The model under review builds one solid part; all positions refer to its coordinate system, in mm. Give positions to 0.01 mm unless a question says otherwise; leave off trailing zeros. Order: outer loops, then holes, each group sorted by start corner. A loop starts at its lowest first (then second) coordinate and runs counter-clockwise, first axis right, second up. Notation, with made-up numbers: (40.5, -20) -> (45.5, -20) arc R18 ccw to (45.5, 9) -> close; hole circle Ø11 at (61, -6). An arc over 180 degrees is marked (long way). Use one line per item in the form item = value.
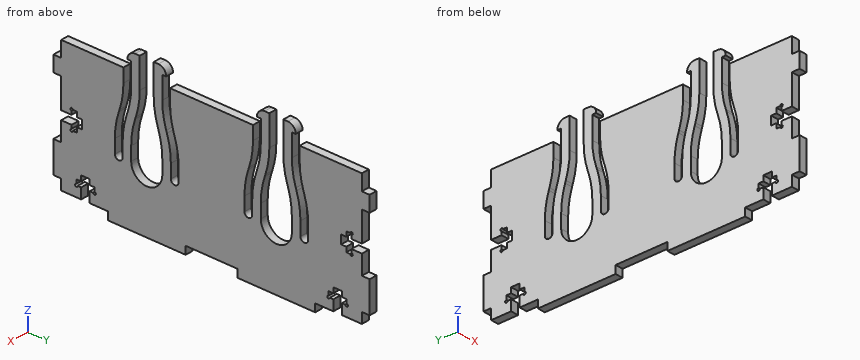
```python
from build123d import *

# Parameters (mm, degrees)
F0_W     = 3
F0_H     = 6
F0_H_2   = 12
F0_W_2   = 30
F0_H_3   = 3
F1_DEPTH = 1.5


# Not quite as in the source:
# - a feature names something its author has since deleted; it is built from what else it names


with BuildPart() as f1:
    # F0 (on Right) → F1 (new body, symmetric)
    with BuildSketch(Plane.YZ):
        with BuildLine():
            Line((50.3, -25), (58, -25))
            Line((58, -25), (58, -21))
            Line((58, -21), (58, -9))
            Line((58, -9), (58, -1.65))
            Line((58, -1.65), (54, -1.65))
            Line((54, -1.65), (54, -3))
            ThreePointArc((54, -3), (54.3535533906, -3.1464466094), (54.5, -3.5))
            ThreePointArc((54.5, -3.5), (54, -4), (53.5, -3.5))
            Line((53.5, -3.5), (52, -3.5))
            Line((52, -3.5), (52, -1.65))
            Line((52, -1.65), (50, -1.65))
            Line((50, -1.65), (50, 1.65))
            Line((50, 1.65), (52, 1.65))
            Line((52, 1.65), (52, 3.5))
            Line((52, 3.5), (53.5, 3.5))
            ThreePointArc((53.5, 3.5), (54, 4), (54.5, 3.5))
            ThreePointArc((54.5, 3.5), (54.3535533906, 3.1464466094), (54, 3))
            Line((54, 3), (54, 1.65))
            Line((54, 1.65), (58, 1.65))
            Line((58, 1.65), (58, 13))
            Line((58, 13), (58, 19))
            Line((58, 19), (58, 25))
            Line((58, 25), (34, 25))
            Line((34, 25), (34, 19.8221099082))
            ThreePointArc((34, 19.8221099082), (34.3801942596, 15.0611112835), (35.5111405269, 10.4207862821))
            Line((35.5111405269, 10.4207862821), (35.7888594731, 9.5792137179))
            ThreePointArc((35.7888594731, 9.5792137179), (36.9198057404, 4.9388887165), (37.3, 0.1778900918))
            Line((37.3, 0.1778900918), (37.3, -5))
            ThreePointArc((37.3, -5), (35.8, -6.5), (34.3, -5))
            Line((34.3, -5), (34.3, 0.1778900918))
            ThreePointArc((34.3, 0.1778900918), (33.9198057404, 4.9388887165), (32.7888594731, 9.5792137179))
            Line((32.7888594731, 9.5792137179), (32.5111405269, 10.4207862821))
            ThreePointArc((32.5111405269, 10.4207862821), (31.3801942596, 15.0611112835), (31, 19.8221099082))
            Line((31, 19.8221099082), (31, 25))
            Line((31, 25), (27.7, 25))
            Line((27.7, 25), (27.7, 19.8221099082))
            ThreePointArc((27.7, 19.8221099082), (28.0801942596, 15.0611112835), (29.2111405269, 10.4207862821))
            Line((29.2111405269, 10.4207862821), (29.4888594731, 9.5792137179))
            ThreePointArc((29.4888594731, 9.5792137179), (30.6198057404, 4.9388887165), (31, 0.1778900918))
            Line((31, 0.1778900918), (31, -5))
            ThreePointArc((31, -5), (25, -11), (19, -5))
            Line((19, -5), (19, 0.1778900918))
            ThreePointArc((19, 0.1778900918), (19.3801942596, 4.9388887165), (20.5111405269, 9.5792137179))
            Line((20.5111405269, 9.5792137179), (20.7888594731, 10.4207862821))
            ThreePointArc((20.7888594731, 10.4207862821), (21.9198057404, 15.0611112835), (22.3, 19.8221099082))
            Line((22.3, 19.8221099082), (22.3, 25))
            Line((22.3, 25), (19, 25))
            Line((19, 25), (19, 19.8221099082))
            ThreePointArc((19, 19.8221099082), (18.6198057404, 15.0611112835), (17.4888594731, 10.4207862821))
            Line((17.4888594731, 10.4207862821), (17.2111405269, 9.5792137179))
            ThreePointArc((17.2111405269, 9.5792137179), (16.0801942596, 4.9388887165), (15.7, 0.1778900918))
            Line((15.7, 0.1778900918), (15.7, -5))
            ThreePointArc((15.7, -5), (14.2, -6.5), (12.7, -5))
            Line((12.7, -5), (12.7, 0.1778900918))
            ThreePointArc((12.7, 0.1778900918), (13.0801942596, 4.9388887165), (14.2111405269, 9.5792137179))
            Line((14.2111405269, 9.5792137179), (14.4888594731, 10.4207862821))
            ThreePointArc((14.4888594731, 10.4207862821), (15.6198057404, 15.0611112835), (16, 19.8221099082))
            Line((16, 19.8221099082), (16, 25))
            Line((16, 25), (-16, 25))
            Line((-16, 25), (-16, 19.8221099082))
            ThreePointArc((-16, 19.8221099082), (-15.6198057404, 15.0611112835), (-14.4888594731, 10.4207862821))
            Line((-14.4888594731, 10.4207862821), (-14.2111405269, 9.5792137179))
            ThreePointArc((-14.2111405269, 9.5792137179), (-13.0801942596, 4.9388887165), (-12.7, 0.1778900918))
            Line((-12.7, 0.1778900918), (-12.7, -5))
            ThreePointArc((-12.7, -5), (-14.2, -6.5), (-15.7, -5))
            Line((-15.7, -5), (-15.7, 0.1778900918))
            ThreePointArc((-15.7, 0.1778900918), (-16.0801942596, 4.9388887165), (-17.2111405269, 9.5792137179))
            Line((-17.2111405269, 9.5792137179), (-17.4888594731, 10.4207862821))
            ThreePointArc((-17.4888594731, 10.4207862821), (-18.6198057404, 15.0611112835), (-19, 19.8221099082))
            Line((-19, 19.8221099082), (-19, 25))
            Line((-19, 25), (-22.3, 25))
            Line((-22.3, 25), (-22.3, 19.8221099082))
            ThreePointArc((-22.3, 19.8221099082), (-21.9198057404, 15.0611112835), (-20.7888594731, 10.4207862821))
            Line((-20.7888594731, 10.4207862821), (-20.5111405269, 9.5792137179))
            ThreePointArc((-20.5111405269, 9.5792137179), (-19.3801942596, 4.9388887165), (-19, 0.1778900918))
            Line((-19, 0.1778900918), (-19, -5))
            ThreePointArc((-19, -5), (-25, -11), (-31, -5))
            Line((-31, -5), (-31, 0.1778900918))
            ThreePointArc((-31, 0.1778900918), (-30.6198057404, 4.9388887165), (-29.4888594731, 9.5792137179))
            Line((-29.4888594731, 9.5792137179), (-29.2111405269, 10.4207862821))
            ThreePointArc((-29.2111405269, 10.4207862821), (-28.0801942596, 15.0611112835), (-27.7, 19.8221099082))
            Line((-27.7, 19.8221099082), (-27.7, 25))
            Line((-27.7, 25), (-31, 25))
            Line((-31, 25), (-31, 19.8221099082))
            ThreePointArc((-31, 19.8221099082), (-31.3801942596, 15.0611112835), (-32.5111405269, 10.4207862821))
            Line((-32.5111405269, 10.4207862821), (-32.7888594731, 9.5792137179))
            ThreePointArc((-32.7888594731, 9.5792137179), (-33.9198057404, 4.9388887165), (-34.3, 0.1778900918))
            Line((-34.3, 0.1778900918), (-34.3, -5))
            ThreePointArc((-34.3, -5), (-35.8, -6.5), (-37.3, -5))
            Line((-37.3, -5), (-37.3, 0.1778900918))
            ThreePointArc((-37.3, 0.1778900918), (-36.9198057404, 4.9388887165), (-35.7888594731, 9.5792137179))
            Line((-35.7888594731, 9.5792137179), (-35.5111405269, 10.4207862821))
            ThreePointArc((-35.5111405269, 10.4207862821), (-34.3801942596, 15.0611112835), (-34, 19.8221099082))
            Line((-34, 19.8221099082), (-34, 25))
            Line((-34, 25), (-58, 25))
            Line((-58, 25), (-58, 19))
            Line((-58, 19), (-58, 13))
            Line((-58, 13), (-58, 1.65))
            Line((-58, 1.65), (-54, 1.65))
            Line((-54, 1.65), (-54, 3))
            ThreePointArc((-54, 3), (-54.3535533906, 3.8535533906), (-53.5, 3.5))
            Line((-53.5, 3.5), (-52, 3.5))
            Line((-52, 3.5), (-52, 1.65))
            Line((-52, 1.65), (-50, 1.65))
            Line((-50, 1.65), (-50, -1.65))
            Line((-50, -1.65), (-52, -1.65))
            Line((-52, -1.65), (-52, -3.5))
            Line((-52, -3.5), (-53.5, -3.5))
            ThreePointArc((-53.5, -3.5), (-54.3535533906, -3.8535533906), (-54, -3))
            Line((-54, -3), (-54, -1.65))
            Line((-54, -1.65), (-58, -1.65))
            Line((-58, -1.65), (-58, -9))
            Line((-58, -9), (-58, -21))
            Line((-58, -21), (-58, -25))
            Line((-58, -25), (-50.3, -25))
            Line((-50.3, -25), (-50.3, -21))
            Line((-50.3, -21), (-51.65, -21))
            ThreePointArc((-51.65, -21), (-52.5035533906, -21.3535533906), (-52.15, -20.5))
            Line((-52.15, -20.5), (-52.15, -19))
            Line((-52.15, -19), (-50.3, -19))
            Line((-50.3, -19), (-50.3, -17))
            Line((-50.3, -17), (-47, -17))
            Line((-47, -17), (-47, -19))
            Line((-47, -19), (-45.15, -19))
            Line((-45.15, -19), (-45.15, -20.5))
            ThreePointArc((-45.15, -20.5), (-44.7964466094, -20.6464466094), (-44.65, -21))
            ThreePointArc((-44.65, -21), (-45.15, -21.5), (-45.65, -21))
            Line((-45.65, -21), (-47, -21))
            Line((-47, -21), (-47, -25))
            Line((-47, -25), (-40, -25))
            Line((-40, -25), (-10, -25))
            Line((-10, -25), (10, -25))
            Line((10, -25), (40, -25))
            Line((40, -25), (47, -25))
            Line((47, -25), (47, -21))
            Line((47, -21), (45.65, -21))
            ThreePointArc((45.65, -21), (44.7964466094, -21.3535533906), (45.15, -20.5))
            Line((45.15, -20.5), (45.15, -19))
            Line((45.15, -19), (47, -19))
            Line((47, -19), (47, -17))
            Line((47, -17), (50.3, -17))
            Line((50.3, -17), (50.3, -19))
            Line((50.3, -19), (52.15, -19))
            Line((52.15, -19), (52.15, -20.5))
            ThreePointArc((52.15, -20.5), (52.5035533906, -20.6464466094), (52.65, -21))
            ThreePointArc((52.65, -21), (52.15, -21.5), (51.65, -21))
            Line((51.65, -21), (50.3, -21))
            Line((50.3, -21), (50.3, -25))
        make_face()
        with Locations((-59.5, 16)):
            Rectangle(F0_W, F0_H)
        with Locations((-59.5, -15)):
            Rectangle(F0_W, F0_H_2)
        with Locations((59.5, 16)):
            Rectangle(F0_W, F0_H)
        with Locations((59.5, -15)):
            Rectangle(F0_W, F0_H_2)
        with Locations((25, -26.5)):
            Rectangle(F0_W_2, F0_H_3)
        with Locations((-25, -26.5)):
            Rectangle(F0_W_2, F0_H_3)
        with BuildLine():
            Line((-31, 28.3), (-31, 25))
            Line((-31, 25), (-27.7, 25))
            Line((-27.7, 25), (-27.7, 31.3))
            Line((-27.7, 31.3), (-29.5, 31.3))
            ThreePointArc((-29.5, 31.3), (-31.6213203436, 30.4213203436), (-32.5, 28.3))
            Line((-32.5, 28.3), (-31, 28.3))
        make_face()
        with BuildLine():
            Line((-22.3, 25), (-19, 25))
            Line((-19, 25), (-19, 28.3))
            Line((-19, 28.3), (-17.5, 28.3))
            ThreePointArc((-17.5, 28.3), (-18.3786796564, 30.4213203436), (-20.5, 31.3))
            Line((-20.5, 31.3), (-22.3, 31.3))
            Line((-22.3, 31.3), (-22.3, 25))
        make_face()
        with BuildLine():
            Line((19, 25), (22.3, 25))
            Line((22.3, 25), (22.3, 31.3))
            Line((22.3, 31.3), (20.5, 31.3))
            ThreePointArc((20.5, 31.3), (18.3786796564, 30.4213203436), (17.5, 28.3))
            Line((17.5, 28.3), (19, 28.3))
            Line((19, 28.3), (19, 25))
        make_face()
        with BuildLine():
            Line((27.7, 25), (31, 25))
            Line((31, 25), (31, 28.3))
            Line((31, 28.3), (32.5, 28.3))
            ThreePointArc((32.5, 28.3), (31.6213203436, 30.4213203436), (29.5, 31.3))
            Line((29.5, 31.3), (27.7, 31.3))
            Line((27.7, 31.3), (27.7, 25))
        make_face()
    extrude(amount=F1_DEPTH, both=True)


solid = f1.part
```
1. For pin 1 Ø1.5 at (x, z) = (-0.5, -3) entering from -Y; pin 2 Ø0.9 at (x, z) = (-0.5, -23.5) entering from +Y; pin 3 Ø1.5 at (x, y) = (0.5, -59.5) entering from -Z, all flat-tipped, find the tip position at first contact; note any pin that passes through.
Values:
pin_1 = -58
pin_2 = 58
pin_3 = -21
2. Add section B-B on y = -5. Give the boundary of the cut face in (x, z).
Values:
outline = (-1.5, -25) -> (1.5, -25) -> (1.5, 25) -> (-1.5, 25) -> close
3. For L1, parallel to Y at x = -0.75, z = -24; L2, parallel to Y at x = 0, z = 27; L3, parallel to Z at x = -0.15, y = -5.5, list the stretches that pass through material, from the lowest coordinate up.
Values:
L1 = -58 to -50.3, -47 to 47, 50.3 to 58
L2 = -31 to -27.7, -22.3 to -19, 19 to 22.3, 27.7 to 31
L3 = -25 to 25
4. Add section A-A on y = -25. Give the boundary of the cut face in (x, z), then the cut area to 3 significant figures.
Values:
outline = (-1.5, -28) -> (1.5, -28) -> (1.5, -11) -> (-1.5, -11) -> close
area = 51.0 mm^2
